Job drawing, mm, ordinate dimensions from the low corner. One solid piece. A direction names the side the tool comes from. Give positions to 0.01 mm unless a question says otherwise; leave off trailing zeros. Write each loop counter-clockwise with the first axis right and the second up, starting at its lowest first coordinate (ties: lowest second). Pieces come first, ordered by that corner, then holes. Notation, with made-up numbers: (16.25, 72.5) - (26.25, 72.5) arc R29 cw to (26.25, 106.5) - close; hole circle Ø10 at (29, -30). An arc over 180 degrees is marked (long way). Put each result on its own line as item: value. Start each with the question number.
1. Wall check: line 1 (Y direction, x = 6.75, z = 6.5); line 2 (Z direction, x = 6.5, y = 1.25); line 3 (X direction, y = 9.75, z = 4.25) (1 decimal). Give the ranges that are in metal, low to high.
2. Cut at C-C on x = 2. List the corners of the cut face in (y, z), and give its area (3 significant figures).
3. Drop flat-ended pins along their axis: pin 1 (1 mm diameter, centred on x = 3, y = 9.5, fed in from -Z); pin 2 (1 mm diameter, centred on x = 3.5, z = 6, fed in from -Y); pin 3 (2 mm diameter, centred on y = 9, z = 3.5, fed in from +X); pin 4 (0.6 mm diameter, centred on y = 11.5, z = 5, fed in from +X). Give the stop position or say it passes through.
4. Cut at B-B on y = 6. List the corners of the cut face in (x, z).
5. Tool access for the marked faces 1, 2, 3 and 4: list every direction of +Z, -Z, +X, -X, +Y, -Y with a clear straight run to the whole face (end or side of a thin tool).
6. Cut at D-D on y = 1. List the corners of the cut face in (x, z).
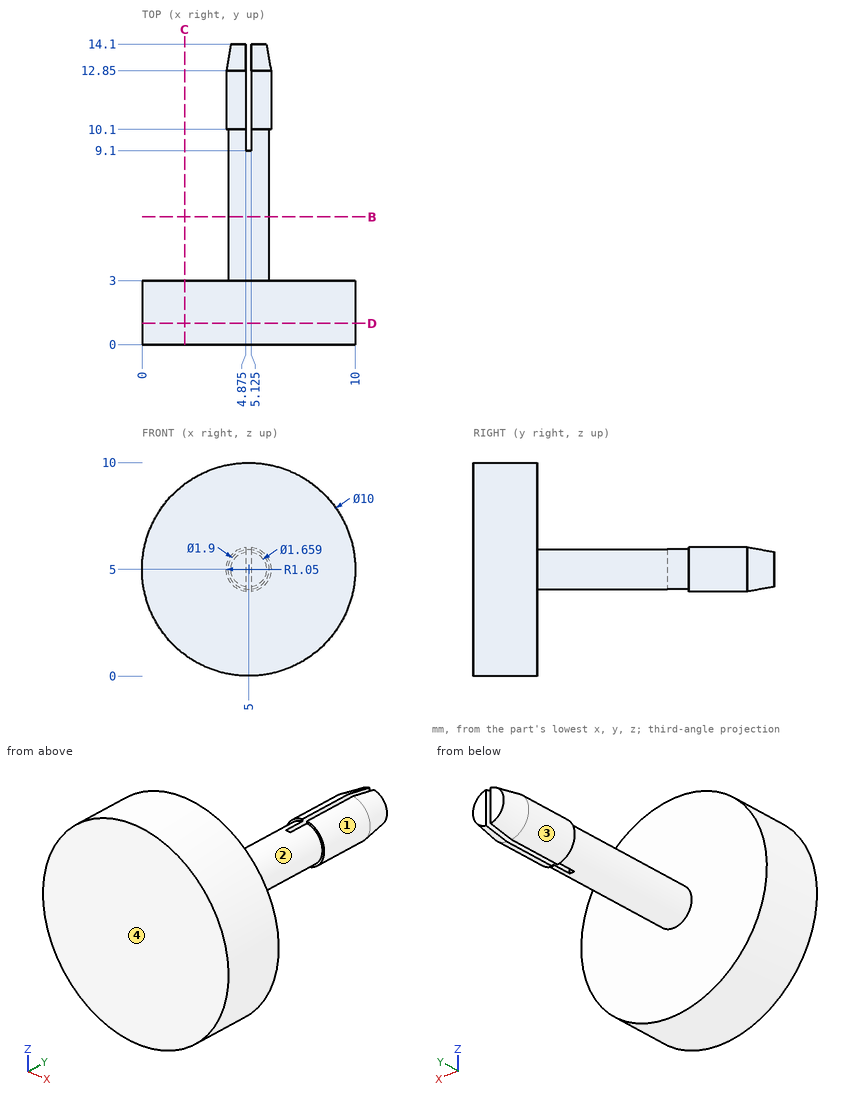
Report:
1. line 1: y = 0 to 3
1. line 2: z = 0.23 to 9.77
1. line 3: x = 4.4 to 4.9, 5.1 to 5.6
2. outline: (0, 1) - (3, 1) - (3, 9) - (0, 9) - close
2. area: 24.0 mm²
3. pin 1: passes through
3. pin 2: stops at y = 0
3. pin 3: stops at x = 5.81
3. pin 4: stops at x = 6.05
4. outline: circle Ø1.9 at (5, 5)
5. face 1: +X, +Y
5. face 2: none
5. face 3: -X, +Y
5. face 4: +Z, -Z, +X, -X, -Y
6. outline: circle Ø10 at (5, 5)
